from build123d import *

# Parameters (mm, degrees)
BOSS_EXTRUDE1_DEPTH = 4
SKETCH2_R           = 1.5875
CUT_EXTRUDE1_DEPTH  = 10
FILLET1_R           = 1
SKETCH3_W           = 4.5
SKETCH3_H           = 0.2
CUT_EXTRUDE2_DEPTH  = 10
FILLET2_R           = 1


with BuildPart() as part:
    # Sketch1 → Boss-Extrude1 (new body, symmetric)
    with BuildSketch(Plane.XY):
        Polygon((0, 0), (6, 0), (9, 3.625), (21, 3.625), (21, 3.825), (8.905909928, 3.825), (5.905909928, 0.2), (0, 0.2), align=None)
    extrude(amount=BOSS_EXTRUDE1_DEPTH, both=True)

    # Sketch2 → Cut-Extrude1 (cut)
    with BuildSketch(Plane(origin=(0, 3.825, 0), x_dir=(1, 0, 0), z_dir=(0, 1, 0))):
        with Locations((17.705909928, 0)):
            Circle(SKETCH2_R)
    extrude(amount=-CUT_EXTRUDE1_DEPTH, mode=Mode.SUBTRACT)

    # Fillet1
    fillet1_edges = [part.edges().sort_by_distance(p)[0] for p in [
        (0, 0.1, -4),
        (21, 3.725, 4),
        (0, 0.1, 4),
        (21, 3.725, -4),
    ]]
    fillet(fillet1_edges, radius=FILLET1_R)

    # Sketch3 → Cut-Extrude2 (cut)
    with BuildSketch(Plane(origin=(0, 0.2, 0), x_dir=(1, 0, 0), z_dir=(0, 1, 0))):
        with Locations((2.25, 0)):
            Rectangle(SKETCH3_W, SKETCH3_H)
    extrude(amount=-CUT_EXTRUDE2_DEPTH, mode=Mode.SUBTRACT)

    # Fillet2
    fillet2_edges = [part.edges().sort_by_distance(p)[0] for p in [
        (5.905909928, 0.2, 0),
        (8.905909928, 3.825, 0),
    ]]
    fillet(fillet2_edges, radius=FILLET2_R)


solid = part.part
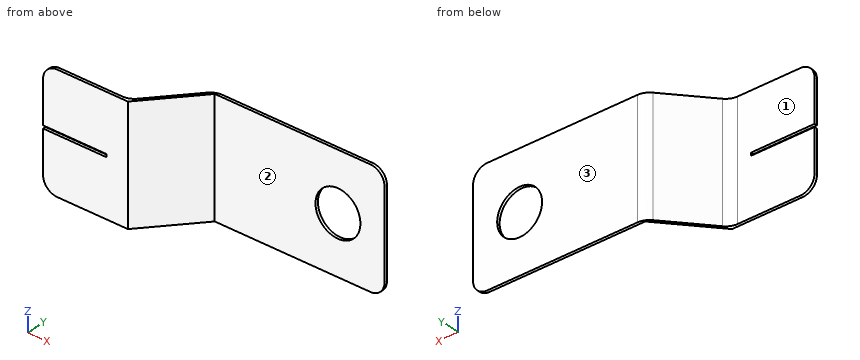
Could you check a few things on this model? Use its own coordinates, in mm. Face numbers are marked on the shaded views. A direction names the side the tool comes from. Round coordinates to 2 decimals unless told otherwise and drop trailing zeros. Write each loop counter-clockwise with the first axis right and the second up, starting at its lowest first coordinate (ties: lowest second). Pieces come first, ordered by that corner, then holes. Notation, with made-up numbers: (65, 14.25) - (107, 14.25) arc R10 ccw to (107, 25.25) - close; hole circle Ø2 at (-25.75, -18). An arc over 180 degrees is marked (long way). Use a Markdown table: item, result.
Q1. I want a section at A-A (z = 2.75). List the corners of the cut face in (x, y) for me (3 decimals).
Output values:
| item | result |
|---|---|
| outline | (0, 0) - (6, 0) - (9, 3.625) - (21, 3.625) - (21, 3.825) - (9.376, 3.825) arc R1 ccw to (8.606, 3.463) - (6.206, 0.562) arc R1 cw to (5.435, 0.2) - (0, 0.2) - close |
Q2. For the marked faces 1, 2 and 3, which set-ups out of +Z, -Z, +X, -X, +Y, -Y let a thin tool reach every point of the face, with its end or its side?
Output values:
| item | result |
|---|---|
| face 1 | +Z, -Z, -X, +Y |
| face 2 | +Z, -Z, +X, -Y |
| face 3 | +Z, -Z, +X, -X, +Y |
Q3. I want a section at B-B (z = -0.75). List the corners of the cut face in (x, y) for me (3 decimals), plus the area to 3 significant figures.
Output values:
| item | result |
|---|---|
| outline | (0, 0) - (6, 0) - (9, 3.625) - (16.307, 3.625) - (16.307, 3.825) - (9.376, 3.825) arc R1 ccw to (8.606, 3.463) - (6.206, 0.562) arc R1 cw to (5.435, 0.2) - (0, 0.2) - close; (19.105, 3.625) - (21, 3.625) - (21, 3.825) - (19.105, 3.825) - close |
| area | 3.98 mm2 |
Q4. For pin 1 (1.6 mm diameter, centred on x = 3.5, z = 0, fed in from +Y); pin 2 (1 mm diameter, centred on x = 7.5, z = -1, fed in from +Y); pin 3 (1.9 mm diameter, centred on x = 17.71, z = 0, fed in from -Y); pin 4 (1.5 mm diameter, centred on y = 0.5, z = -3, fed in from +X), each with a flat end and sliding along its axis, tell me the tip position at first contact or that it passes through.
Output values:
| item | result |
|---|---|
| pin 1 | y = 0.2 |
| pin 2 | y = 2.73 |
| pin 3 | through |
| pin 4 | x = 7.03 |
Q5. Please list where these lines run through material, in increasing order: L1, parallel to Y at x = 20, z = -1.75 (3 decimals); L2, parallel to Y at x = 5.5, z = 1.25; L3, parallel to X at y = 3.7, z = 0.
Output values:
| item | result |
|---|---|
| L1 | 3.625 to 3.825 |
| L2 | 0 to 0.2 |
| L3 | 8.89 to 16.12, 19.29 to 21 |
Q6. I want a section at C-C (x = 14). List the corners of the cut face in (y, z) for me (3 decimals).
Output values:
| item | result |
|---|---|
| outline | (3.625, -4) - (3.825, -4) - (3.825, 4) - (3.625, 4) - close |
